Verification items for the finished model (mm, model axes). A direction names the side the tool comes from. Give positions to 0.01 mm unless a question says otherwise; leave off trailing zeros. Loops run counter-clockwise (first coordinate to the right, second up) from the corner with the lowest first, then second, coordinate; pieces in that order, holes last. Notation, with made-up numbers: M 41,-27.75 L 59,-27.75 A23 ccw 59,-17.75 Z; hole C 9.25,7.25 d4. An arc over 180 degrees is marked long. Answer in a Markdown table with one row per item.
```python
from build123d import *

# Parameters (mm, degrees)
BOSS_EXTRUDE1_DEPTH = 5
BOSS_EXTRUDE2_DEPTH = 10
BOSS_EXTRUDE3_DEPTH = 5
CUT_EXTRUDE1_DEPTH  = 5
CUT_EXTRUDE2_DEPTH  = 1
CIRPATTERN1_COUNT   = 25
CIRPATTERN1_ANGLE   = 120
CUT_EXTRUDE3_DEPTH  = 16
CHAMFER1_SIZE       = 0.25


with BuildPart() as part:
    # Sketch1 → Boss-Extrude1 (new body)
    with BuildSketch(Plane(origin=(0, 0, 0), x_dir=(1, 0, 0), z_dir=(0, 1, 0))):
        with BuildLine():
            Line((-69.75, 120.810543828), (-82.5, 142.894191624))
            ThreePointArc((-82.5, 142.894191624), (82.5, 142.894191624), (165, 0))
            Line((165, 0), (139.5, 0))
            ThreePointArc((139.5, 0), (69.75, 120.810543828), (-69.75, 120.810543828))
        make_face()
    extrude(amount=BOSS_EXTRUDE1_DEPTH)

    # Sketch2 → Boss-Extrude2 (add)
    with BuildSketch(Plane(origin=(0, 5, 0), x_dir=(1, 0, 0), z_dir=(0, 1, 0))):
        with BuildLine():
            Line((-72.25, 125.140670847), (-69.75, 120.810543828))
            ThreePointArc((-69.75, 120.810543828), (69.75, 120.810543828), (139.5, 0))
            Line((139.5, 0), (144.5, 0))
            ThreePointArc((144.5, 0), (72.25, 125.140670847), (-72.25, 125.140670847))
        make_face()
    extrude(amount=BOSS_EXTRUDE2_DEPTH)

    # Sketch3 → Boss-Extrude3 (add)
    with BuildSketch(Plane(origin=(0, 5, 0), x_dir=(1, 0, 0), z_dir=(0, 1, 0))):
        with BuildLine():
            Line((-71.88125, 124.501977112), (-73.88125, 127.966078727))
            Line((-73.88125, 127.966078727), (-75.613300808, 126.966078727))
            ThreePointArc((-75.613300808, 126.966078727), (-78.430339344, 123.030259693), (-73.613300808, 123.501977112))
            Line((-73.613300808, 123.501977112), (-71.88125, 124.501977112))
        make_face()
        with BuildLine():
            Line((-78.14375, 135.348945294), (-80.14375, 138.813046909))
            Line((-80.14375, 138.813046909), (-81.875800808, 137.813046909))
            ThreePointArc((-81.875800808, 137.813046909), (-84.692839344, 133.877227875), (-79.875800808, 134.348945294))
            Line((-79.875800808, 134.348945294), (-78.14375, 135.348945294))
        make_face()
    extrude(amount=-BOSS_EXTRUDE3_DEPTH)

    # Sketch4 → Cut-Extrude1 (cut)
    with BuildSketch(Plane(origin=(0, 0, 0), x_dir=(1, 0, 0), z_dir=(0, 1, 0))):
        with BuildLine():
            Line((156.6375, 1.962821416), (156.6375, 0))
            Line((156.6375, 0), (160.8375, 0))
            Line((160.8375, 0), (160.8375, 1.962821416))
            ThreePointArc((160.8375, 1.962821416), (158.7375, 6.507536453), (156.6375, 1.962821416))
        make_face()
        with BuildLine():
            Line((143.6625, 1.962821416), (143.6625, 0))
            Line((143.6625, 0), (147.8625, 0))
            Line((147.8625, 0), (147.8625, 1.962821416))
            ThreePointArc((147.8625, 1.962821416), (145.7625, 6.507536453), (143.6625, 1.962821416))
        make_face()
    extrude(amount=CUT_EXTRUDE1_DEPTH, mode=Mode.SUBTRACT)

    # Sketch5 → Cut-Extrude2 (cut)
    with BuildSketch(Plane(origin=(0, 15, 0), x_dir=(1, 0, 0), z_dir=(0, 1, 0))):
        Polygon((-72.659271704, 126.849550232), (-68.346968319, 119.380421672), (-69.212993723, 118.880421672), (-73.606467483, 126.490141447), align=None)
    cut_extrude2 = extrude(amount=-CUT_EXTRUDE2_DEPTH, mode=Mode.SUBTRACT)

    # CirPattern1: Cut-Extrude2 ×25 about axis
    cirpattern1_axis = Axis((0, 0, 0), (0, -1, 0))
    for i in range(1, CIRPATTERN1_COUNT):
        add(cut_extrude2.rotate(cirpattern1_axis, i * CIRPATTERN1_ANGLE / (CIRPATTERN1_COUNT - 1)), mode=Mode.SUBTRACT)

    # Sketch6 → Cut-Extrude3 (cut, through all)
    with BuildSketch(Plane(origin=(0, 15, 0), x_dir=(1, 0, 0), z_dir=(0, 1, 0))):
        Polygon((134.134253662, 0), (167.805161023, 0), (167.805161023, 0.1), (133.91215317, 0.1), align=None)
    extrude(amount=-CUT_EXTRUDE3_DEPTH, mode=Mode.SUBTRACT)

    # Chamfer1
    chamfer1_edges = [part.edges().sort_by_distance(p)[0] for p in [
        (-81.009775404, 5, -138.313046909),
        (-84.692839344, 5, -133.877227875),
        (-79.009775404, 5, -134.848945294),
        (-74.747275404, 5, -127.466078727),
        (-78.430339344, 5, -123.030259693),
        (-72.747275404, 5, -124.001977112),
    ]]
    chamfer(chamfer1_edges, length=CHAMFER1_SIZE)


solid = part.part
```
Item 1: Sectioned sample at B-B (y = 7.75). Record the cut outline in (x, z), and give its area (3 significant figures).
Reported:
| item | result |
|---|---|
| outline | M -72.25,-125.14 A144.5 ccw 144.5,-0.1 L 139.5,-0.1 A139.5 cw -69.75,-120.81 Z |
| area | 1,490 mm^2 |
Item 2: Go/stop test with flat-tipped pins: pin 1 (4 mm diameter, centred on y = 10, z = -95.5, fed in from -X); pin 2 (5 mm diameter, centred on x = 46, y = 7, fed in from -Z); pin 3 (2 mm diameter, centred on y = 2.5, z = -138, fed in from -X). Record where each tip stops, or that it passes through.
Reported:
| item | result |
|---|---|
| pin 1 | stops at x = 99.77 |
| pin 2 | stops at z = -158.89 |
| pin 3 | stops at x = -84.35 |
Item 3: Sectioned sample at D-D (z = -155). Record the cut outline in (x, y).
Reported:
| item | result |
|---|---|
| outline | M -56.57,0 L 56.57,0 L 56.57,5 L -56.57,5 Z |
Item 4: Release check for a two-part mould opening along Z. For faces 1 (the conical face through (-78.36, 4.88, -123.17)), 2 (the flat face through (76, 15, -120)), 3 (the cylindrical face through (158.825, 2.465, -6.506)), 4 (the flat face through (142, 7, -0.1)) record: released by +Z, released by -Z, zero draft, split by the parting line, or undercut.
Reported:
| item | result |
|---|---|
| face 1 | undercut |
| face 2 | zero draft |
| face 3 | undercut |
| face 4 | released by +Z |
Item 5: Sectioned sample at C-C (x = -5). Record the cut outline in (y, z), and give its area (3 significant figures).
Reported:
| item | result |
|---|---|
| outline | M 0,-164.92 L 5,-164.92 L 5,-144.41 L 15,-144.41 L 15,-139.41 L 0,-139.41 Z |
| area | 178 mm^2 |
Item 6: Scan lines: L1, parallel to X at y = 1.3, z = -3.75; L2, parallel to X at y = 7, z = -127.5; L3, parallel to Y at x = 151, z = -57.5. Record each from-to range of solid material in increasing order. Write a range as [from, to].
Reported:
| item | result |
|---|---|
| L1 | x = [139.45, 143], [148.52, 155.98], [161.5, 164.96] |
| L2 | x = [-68, -56.6], [56.6, 68] |
| L3 | y = [0, 5] |
Item 7: Tool access check on faces 5 (the flat face through (-43, 15, -135)), 6 (the flat face through (58, 5, -138)). Record the directions out of +Z, -Z, +X, -X, +Y, -Y that give a thin tool (end or side, any length) a straight path to the whole face; none if there is none.
Reported:
| item | result |
|---|---|
| face 5 | +Z, -Z, +X, -X, +Y |
| face 6 | -Z, +Y |
Item 8: Sectioned sample at A-A (z = -17.5). Record the cut outline in (x, y).
Reported:
| item | result |
|---|---|
| outline | M 138.4,0 L 164.07,0 L 164.07,5 L 143.44,5 L 143.44,15 L 138.4,15 Z |
